Part model, mm, in its own coordinate system. A direction names the side the tool comes from. Give positions to 0.01 mm unless a question says otherwise; leave off trailing zeros. Write each loop counter-clockwise with the first axis right and the second up, starting at its lowest first coordinate (ties: lowest second). Pieces come first, ordered by that corner, then holes.
Autodesk Inventor part; units mm, degrees
ref_plane "YZ Plane" through (0, 0, 0) normal (1, 0, 0) x (0, 1, 0)
ref_plane "XZ Plane" through (0, 0, 0) normal (0, 1, 0) x (-1, 0, 0)
ref_plane "XY Plane" through (0, 0, 0) normal (0, 0, 1) x (1, 0, 0)
sketch "main" plane through (0, 0, 0) normal (0, 0, 1) x (1, 0, 0)
  arc A0 (11.6558, 28.6956) -> (2.6985, 37.6987) centre (7.1771, 33.1971) ccw
  circle A1 centre (-10.8061, -10.1403) radius 2.1844
  arc A2 (-17.1561, -10.1402) -> (-4.4561, -10.1282) centre (-10.8061, -10.1403) ccw
  line L0 (2.6985, 37.6987) -> (-15.2847, 19.807)
  circle A3 centre (-1.8258, 24.24) radius 2.1844
  line L1 (11.6558, 28.6956) -> (-2.5847, 14.5275)
  line L2 (-10.8061, 15.2597) -> (27.2939, 15.2597) construction
  circle A4 centre (-10.8061, 2.5597) radius 2.1844
  line L3 (-4.4561, -10.1282) -> (-4.4561, 10.026)
  arc A5 (-2.5847, 14.5275) -> (-4.4561, 10.026) centre (1.8939, 10.026) ccw
  line L4 (-17.1561, -10.1402) -> (-17.1561, 15.3055)
  circle A6 centre (-10.8061, 15.2597) radius 2.0955
  arc A7 (-15.2847, 19.807) -> (-17.1561, 15.3055) centre (-10.8061, 15.3055) ccw
  line L5 (7.1771, 37.6513) -> (11.6313, 33.1971)
  line L6 (11.6313, 33.1971) -> (7.1771, 28.7429)
  line L7 (7.1771, 28.7429) -> (2.7229, 33.1971)
  line L8 (2.7229, 33.1971) -> (7.1771, 37.6513)
  line L9 (7.1771, 37.6513) -> (7.1771, 28.7429) construction
  line L10 (11.6313, 33.1971) -> (2.7229, 33.1971) construction
  line L11 (7.1771, 37.6513) -> (13.4763, 37.6513) construction
  point P0 (0.9467, 22.1756)
  point P1 (5.5442, 34.8331)
  point P2 (8.7899, 34.8537)
  point P3 (5.5158, 31.5901)
  dimension "d0" = 12.7
  dimension "d5" = 12.7
  dimension "d6" = 6.35
  dimension "d9" = 6.2992
  dimension "d10" = 45
  dimension "d11" = 6.2992
sketch "Sketch1" plane through (0, 0, 0) normal (0, 1, 0) x (-1, 0, 0)
  arc A0 (22.4619, 13.4358) -> (13.5045, 22.439) centre (17.9832, 17.9374) ccw
  circle A1 centre (0, -25.4) radius 2.1844
  arc A2 (-6.35, -25.4) -> (6.35, -25.3879) centre (0, -25.4) ccw
  line L0 (13.5045, 22.439) -> (-4.4786, 4.5473)
  circle A3 centre (8.9803, 8.9803) radius 2.1844
  line L1 (22.4619, 13.4358) -> (8.2213, -0.7322)
  line L2 (0, 0) -> (38.1, 0) construction
  circle A4 centre (0, -12.7) radius 2.1844
  line L3 (6.35, -25.3879) -> (6.35, -5.2338)
  arc A5 (8.2213, -0.7322) -> (6.35, -5.2338) centre (12.7, -5.2338) ccw
  line L4 (-6.35, -25.4) -> (-6.35, 0.0457)
  circle A6 centre (0, 0) radius 2.0955
  arc A7 (-4.4786, 4.5473) -> (-6.35, 0.0457) centre (0, 0.0457) ccw
  line L5 (17.9832, 22.3916) -> (22.4374, 17.9374)
  line L6 (22.4374, 17.9374) -> (17.9832, 13.4832)
  line L7 (17.9832, 13.4832) -> (13.529, 17.9374)
  line L8 (13.529, 17.9374) -> (17.9832, 22.3916)
  line L9 (17.9832, 22.3916) -> (17.9832, 13.4832) construction
  line L10 (22.4374, 17.9374) -> (13.529, 17.9374) construction
  line L11 (17.9832, 22.3916) -> (24.2824, 22.3916) construction
extrude "Extrusion1" add sketch "Sketch1" along normal blind 1.5875
properties part number "gusset" material "Acetal Resin, White"
1) Saw through at C-C (y = 1.2). Write the cut outline in (x, z).
Check result:
outline: (-22.46, 13.44) - (-8.22, -0.73) arc R6.35 cw to (-6.35, -5.23) - (-6.35, -25.39) arc R6.35 ccw to (6.35, -25.4) - (6.35, 0.05) arc R6.35 ccw to (4.48, 4.55) - (-13.5, 22.44) arc R6.35 ccw to start; hole (-22.44, 17.94) - (-17.98, 13.48) - (-13.53, 17.94) - (-17.98, 22.39) - close; hole circle Ø4.37 at (-8.98, 8.98); hole circle Ø4.37 at (0, -25.4); hole circle Ø4.37 at (0, -12.7); hole circle Ø4.19 at (0, 0)
2) Saw through at D-D (x = 1.5). Write the cut outline in (y, z), and give its area (3 significant figures).
Check result:
outline: (0, -31.57) - (1.59, -31.57) - (1.59, -26.99) - (0, -26.99) - close; (0, -23.81) - (1.59, -23.81) - (1.59, -14.29) - (0, -14.29) - close; (0, -11.11) - (1.59, -11.11) - (1.59, -1.46) - (0, -1.46) - close; (0, 1.46) - (1.59, 1.46) - (1.59, 7.51) - (0, 7.51) - close
area: 47.3 mm2
3) Flat gauge pins, fed straight in: P1, Ø3.5, axis at x = -8.98, z = 8.98, coming from the -Y side; P2, Ø0.5, axis at y = 0.5, z = -19, coming from the -X side. Where does each tip first touch, or does it go through?
Check result:
P1: passes through
P2: stops at x = -6.35
4) 3-axis set-ups, long thin cutter, end or side, ignore diameter. For faces 1 (the flat face through (-6.35, 1, -15)), 2 (the flat face through (-15.787, 0.783, 15.679)), 3 (the flat face through (-5, 1.588, -3)): which of +Z, -Z, +X, -X, +Y, -Y reach the whole face in a straight line?
Check result:
face 1: -Z, -X, +Y, -Y
face 2: +Y, -Y
face 3: +Z, -Z, +X, -X, +Y
5) Saw through at A-A (z = -12.7). Write the cut outline in (x, y).
Check result:
outline: (-6.35, 0) - (-2.18, 0) - (-2.18, 1.59) - (-6.35, 1.59) - close; (2.18, 0) - (6.35, 0) - (6.35, 1.59) - (2.18, 1.59) - close
6) Drill centre lines: L1, parallel to Z at x = 0, y = 0.5; L2, parallel to X at y = 1.15, z = -20; L3, parallel to X at y = 0.3, z = 7. Where is each one in solid material? Low to high.
Check result:
L1: z = -31.75 to -27.58, -23.22 to -14.88, -10.52 to -2.1, 2.1 to 9
L2: x = -6.35 to 6.35
L3: x = -15.99 to -9.9, -8.06 to 2.01
7) Mould opens along X. For faces 4 (the cylindrical face through (0.284, 0.783, -27.566)), 5 (the cylindrical face through (-22.4, 0.8, 22.5)), 6 (the flat face through (-20.179, 0.783, 20.196)), 7 (the cylindrical face through (5.877, 0.783, 2.451)) say: +X half, -X half, draft (parallel to the pull), parting line (faces both ways), or undercut.
Check result:
face 4: undercut
face 5: parting line
face 6: undercut
face 7: +X half
8) Saw through at B-B (x = -14.5). Write the cut outline in (y, z), and give its area (3 significant figures).
Check result:
outline: (0, 5.51) - (1.59, 5.51) - (1.59, 16.97) - (0, 16.97) - close; (0, 18.91) - (1.59, 18.91) - (1.59, 23.25) - (0, 23.25) - close
area: 25.1 mm2
